Autodesk Inventor part; units mm, degrees
ref_plane "YZ Plane" through (0, 0, 0) normal (1, 0, 0) x (0, 1, 0)
ref_plane "XZ Plane" through (0, 0, 0) normal (0, 1, 0) x (-1, 0, 0)
ref_plane "XY Plane" through (0, 0, 0) normal (0, 0, 1) x (1, 0, 0)
sketch "Sketch1" plane through (0, 0, 0) normal (0, 0, 1) x (1, 0, 0)
  circle A0 centre (-17.8844, -9.45) radius 1.4 construction
  line L0 (-22, -13.95) -> (-22, -7.7794) construction
  line L1 (5.75, -13.95) -> (-22, -13.95) construction
  line L2 (5.75, 0) -> (5.75, -13.95) construction
  line L3 (5.75, 0) -> (0, 0) construction
  line L4 (0, 0) -> (0, -7.7794) construction
  line L5 (-14.8242, -7.7794) -> (0, -7.7794) construction
  line L6 (-14.8242, -4.7794) -> (-14.8242, -7.7794) construction
  line L7 (-21.3713, -4.7794) -> (-14.8242, -4.7794) construction
  line L8 (-21.3713, -7.7794) -> (-21.3713, -4.7794) construction
  line L9 (-22, -7.7794) -> (-21.3713, -7.7794) construction
  circle A1 centre (-17.8844, 25.55) radius 1.4 construction
  line L10 (-22, 23.8794) -> (-22, 30.05) construction
  line L11 (-22, 23.8794) -> (-21.3713, 23.8794) construction
  line L12 (-21.3713, 20.8794) -> (-21.3713, 23.8794) construction
  line L13 (-14.8242, 20.8794) -> (-21.3713, 20.8794) construction
  line L14 (-14.8242, 23.8794) -> (-14.8242, 20.8794) construction
  line L15 (-14.8242, 23.8794) -> (0, 23.8794) construction
  line L16 (0, 16.1) -> (0, 23.8794) construction
  line L17 (5.75, 16.1) -> (0, 16.1) construction
  line L18 (5.75, 16.1) -> (5.75, 30.05) construction
  line L19 (5.75, 30.05) -> (-22, 30.05) construction
  line L20 (-23.6597, 10.55) -> (-31.2138, 10.55) construction
  arc A2 (-23.6597, 5.55) -> (-23.6597, 10.55) centre (-23.6597, 8.05) ccw construction
  line L21 (-31.2138, 5.55) -> (-23.6597, 5.55) construction
  line L22 (-31.2138, 5.55) -> (-31.2138, -1.8612) construction
  line L23 (-19.2138, -1.8612) -> (-31.2138, -1.8612) construction
  line L24 (-19.2138, 17.9612) -> (-19.2138, -1.8612) construction
  line L25 (-31.2138, 17.9612) -> (-19.2138, 17.9612) construction
  line L26 (-31.2138, 17.9612) -> (-31.2138, 10.55) construction
  line L27 (5.75, 30.05) -> (-34.7444, 30.05)
  line L28 (-34.7444, 30.05) -> (-34.7444, -13.95)
  line L29 (-34.7444, -13.95) -> (5.75, -13.95)
  line L30 (5.75, -13.95) -> (5.75, 30.05)
  circle A3 centre (-17.8844, 25.55) radius 1.4
  circle A4 centre (-17.8844, -9.45) radius 1.4
  line L31 (-23.6597, 8.05) -> (-27.2138, 8.05) construction
  line L32 (-23.6597, 12.05) -> (-27.2138, 12.05)
  line L33 (-27.2138, 4.05) -> (-23.6597, 4.05)
  arc A5 (-23.6597, 4.05) -> (-23.6597, 12.05) centre (-23.6597, 8.05) ccw
  arc A6 (-27.2138, 12.05) -> (-27.2138, 4.05) centre (-27.2138, 8.05) ccw
  point P0 (-25.4367, 8.05)
  dimension "d2" = 8
extrude "Extrusion1" add sketch "Sketch1" along normal blind 5.5
properties part number "plate"
Could you check a few things on this model? Use its own coordinates, in mm. A direction names the side the tool comes from. Give positions to 0.01 mm unless a question says otherwise; leave off trailing zeros. Loops run counter-clockwise (first coordinate to the right, second up) from the corner with the lowest first, then second, coordinate; pieces in that order, holes last. Notation, with made-up numbers: (49.5, 57) -> (106.5, 57) arc R26 cw to (106.5, 84) -> close; hole circle Ø11 at (47.25, 24). An arc over 180 degrees is marked (long way). Return JSON: item names as keys, results as strings.
Item 1: If we section it at B-B on z = 1.7: List the corners of the cut face in (x, y) for me.
Geometry results:
{"outline": "(-34.74, -13.95) -> (5.75, -13.95) -> (5.75, 30.05) -> (-34.74, 30.05) -> close; hole (-27.21, 4.05) -> (-23.66, 4.05) arc R4 ccw to (-23.66, 12.05) -> (-27.21, 12.05) arc R4 ccw to start; hole circle Ø2.8 at (-17.88, -9.45); hole circle Ø2.8 at (-17.88, 25.55)"}
Item 2: We'd pull the mould along Y, two halves only. Please class faces 3 (the flat face through (-14, 30.05, 3)), 4 (the cylindrical face through (-31.213, 7.962, 2.712)), 5 (the flat face through (-15, -13.95, 3)): +Y half, -Y half, draft (parallel to the pull), parting line (faces both ways), or undercut.
Geometry results:
{"face 3": "+Y half", "face 4": "undercut", "face 5": "-Y half"}
Item 3: Which directions (+Z, -Z, +X, -X, +Y, -Y) give clear straight access to the entire face, cutting with the end or side of a thin tool? Please do faces 1 (the cylindrical face through (-19.66, 8.14, 2.71)), 2 (the flat face through (-15, 8, 5.5)).
Geometry results:
{"face 1": "+Z, -Z", "face 2": "+Z, +X, -X, +Y, -Y"}
Item 4: I'm going to push a flat-ended pin straight in: pin 1 (2 mm diameter, centred on x = -17.88, y = 25.55, fed in from -Z). Where does the tip first touch, or does it pass through?
Geometry results:
{"pin 1": "passes through"}
Item 5: If we section it at C-C on y = -9.45: List the corners of the cut face in (x, z) for me.
Geometry results:
{"outline": "(-34.74, 0) -> (-19.28, 0) -> (-19.28, 5.5) -> (-34.74, 5.5) -> close; (-16.48, 0) -> (5.75, 0) -> (5.75, 5.5) -> (-16.48, 5.5) -> close"}
Item 6: I need wall thicknesses on L1, parallel to Y at x = -26, z = 5.2; L2, parallel to X at y = 25, z = 3.65; L3, parallel to X at y = -8.5, z = 3.95. Which ranges of each line are inside material? Lowest first, please. Write a range as from..to.
Geometry results:
{"L1": "y = -13.95..4.05, 12.05..30.05", "L2": "x = -34.74..-19.17, -16.6..5.75", "L3": "x = -34.74..-18.91, -16.86..5.75"}
Item 7: If we section it at A-A on y = 8.05: List the corners of the cut face in (x, z) for me, plus the area to 3 significant figures.
Geometry results:
{"outline": "(-34.74, 0) -> (-31.21, 0) -> (-31.21, 5.5) -> (-34.74, 5.5) -> close; (-19.66, 0) -> (5.75, 0) -> (5.75, 5.5) -> (-19.66, 5.5) -> close", "area": "159 mm²"}
